```python
from build123d import *

# Parameters (mm, degrees)
SKETCH1_W               = 34.29
SKETCH1_H               = 25.4
BOSS_EXTRUDE1_DEPTH     = 2.54
SKETCH3_W               = 49.53
SKETCH3_H               = 6.35
BOSS_EXTRUDE2_DEPTH     = 3.81
CUT_EXTRUDE1_DEPTH      = 50.415894204
CUT_EXTRUDE1_DEPTH_BACK = 50.415894204
SKETCH2_R               = 1.778
SKETCH5_W               = 7.62
SKETCH5_H               = 6.35
BOSS_EXTRUDE3_DEPTH     = 15.24
BOSS_EXTRUDE4_REACH     = 53.321
SKETCH6_W               = 7.62
SKETCH6_H               = 5.08
SKETCH7_R               = 2.04
SKETCH7_R_2             = 2.039999984
CUT_EXTRUDE2_DEPTH      = 53.578613523
SKETCH9_W               = 2.794
SKETCH9_H               = 12.699691263
CUT_EXTRUDE3_DEPTH      = 58.711684259


with BuildPart() as part:
    # Sketch1 → Boss-Extrude1 (new body)
    with BuildSketch(Plane.XY):
        with Locations((17.145, 12.7)):
            Rectangle(SKETCH1_W, SKETCH1_H)
    extrude(amount=BOSS_EXTRUDE1_DEPTH)

    # Sketch3 → Boss-Extrude2 (add)
    with BuildSketch(Plane(origin=(0, 0, 0), x_dir=(-1, 0, 0), z_dir=(0, 0, -1))):
        with Locations((-17.145, 22.225)):
            Rectangle(SKETCH3_W, SKETCH3_H)
        with Locations((-17.145, 3.175)):
            Rectangle(SKETCH3_W, SKETCH3_H)
    extrude(amount=BOSS_EXTRUDE2_DEPTH)

    # Sketch2 → Cut-Extrude1 (cut, two sides: drawn at the far end of the back side and taken through both)
    with BuildSketch(Plane.XY.offset(2.54).offset(-CUT_EXTRUDE1_DEPTH_BACK)):
        with Locations((3.429, 22.606)):
            Circle(SKETCH2_R)
        with Locations((29.845, 22.86)):
            Circle(SKETCH2_R)
        with Locations((3.429, 2.794)):
            Circle(SKETCH2_R)
        with Locations((29.845, 2.286)):
            Circle(SKETCH2_R)
    extrude(amount=CUT_EXTRUDE1_DEPTH + CUT_EXTRUDE1_DEPTH_BACK, mode=Mode.SUBTRACT)

    # Sketch5 → Boss-Extrude3 (add)
    with BuildSketch(Plane.XY):
        with Locations((-3.81, 22.225)):
            Rectangle(SKETCH5_W, SKETCH5_H)
        with Locations((38.1, 22.225)):
            Rectangle(SKETCH5_W, SKETCH5_H)
        with Locations((38.1, 3.175)):
            Rectangle(SKETCH5_W, SKETCH5_H)
        with Locations((-3.81, 3.175)):
            Rectangle(SKETCH5_W, SKETCH5_H)
    extrude(amount=BOSS_EXTRUDE3_DEPTH)

    # Sketch6 → Boss-Extrude4 (add, up to next)
    with BuildSketch(Plane.XZ, mode=Mode.PRIVATE) as boss_extrude4_sk1:
        with Locations((-3.81, 12.7)):
            Rectangle(SKETCH6_W, SKETCH6_H)
    boss_extrude4_tool1 = extrude(boss_extrude4_sk1.sketch, amount=-BOSS_EXTRUDE4_REACH, mode=Mode.PRIVATE) - part.part
    # Sketch6 → Boss-Extrude4 (add, up to next)
    with BuildSketch(Plane.XZ, mode=Mode.PRIVATE) as boss_extrude4_sk2:
        with Locations((38.1, 12.7)):
            Rectangle(SKETCH6_W, SKETCH6_H)
    boss_extrude4_tool2 = extrude(boss_extrude4_sk2.sketch, amount=-BOSS_EXTRUDE4_REACH, mode=Mode.PRIVATE) - part.part
    add(boss_extrude4_tool1.solids().sort_by_distance((-3.81, 0, 12.7))[0])
    add(boss_extrude4_tool2.solids().sort_by_distance((38.1, 0, 12.7))[0])

    # Sketch7 → Cut-Extrude2 (cut, through all)
    with BuildSketch(Plane.XY.offset(15.24)):
        with Locations((38.1, 3.81)):
            Circle(SKETCH7_R)
        with Locations((38.1, 21.59)):
            Circle(SKETCH7_R_2)
        with Locations((-3.81, 3.81)):
            Circle(SKETCH7_R_2)
        with Locations((-3.81, 21.59)):
            Circle(SKETCH7_R_2)
    extrude(amount=-CUT_EXTRUDE2_DEPTH, mode=Mode.SUBTRACT)

    # Sketch9 → Cut-Extrude3 (cut, through all)
    with BuildSketch(Plane.ZY.offset(7.62)):
        with Locations((11.557, 12.700154369)):
            Rectangle(SKETCH9_W, SKETCH9_H)
    extrude(amount=-CUT_EXTRUDE3_DEPTH, mode=Mode.SUBTRACT)


solid = part.part
```
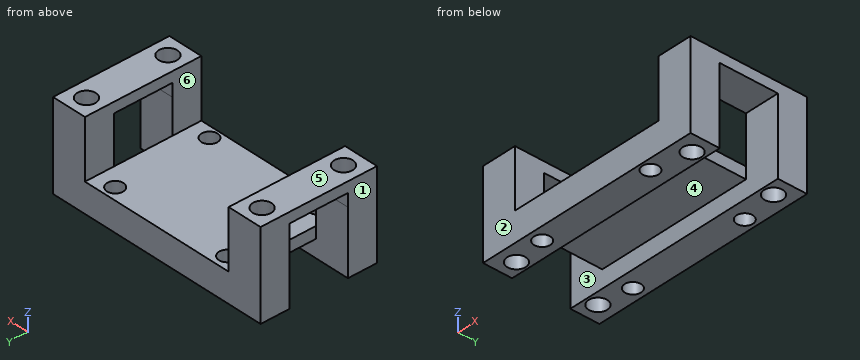
Check sheet for the modelled part. Datum: model origin and axes. Units: mm. Face numbers are marked on the shaded views. A direction names the side the tool comes from. Give positions to 0.01 mm unless a question says otherwise; leave off trailing zeros. Order: outer loops, then holes, each group sorted by start corner. A loop starts at its lowest first (then second) coordinate and runs counter-clockwise, first axis right, second up. Notation, with made-up numbers: (14, 75.25) -> (44, 75.25) arc R12 cw to (44, 79.25) -> close; hole circle Ø5 at (0.5, 84). An arc over 180 degrees is marked (long way). Return JSON: item names as keys, results as strings.
1. Go/stop test with flat-tipped pins: P1, Ø3, axis at y = 14, z = 1, coming from the +X side; P2, Ø0.8, axis at y = 10, z = 1, coming from the -X side; P3, Ø8, axis at x = 20, y = 7.5, coming from the +Z side. Record where each tip stops, or that it passes through.
From the geometry:
{"P1": "x = 34.29", "P2": "x = 0", "P3": "z = 2.54"}
2. Cross-section at B-B, the plane x = -3.81. Count the separate pieces of the cut face and the enclosed holes in it, plus the area to 3 significant figures.
From the geometry:
{"separate pieces": "3", "enclosed holes": "0", "area": "116 mm^2"}
3. Cross-section at C-C, the plane y = 17.75. Record the cut outline in (x, z).
From the geometry:
{"outline": "(-7.62, 12.95) -> (0, 12.95) -> (0, 15.24) -> (-7.62, 15.24) -> close; (0, 0) -> (34.29, 0) -> (34.29, 2.54) -> (0, 2.54) -> close; (34.29, 12.95) -> (41.91, 12.95) -> (41.91, 15.24) -> (34.29, 15.24) -> close"}
4. Mould release check, pull along Y, two halves, no side actions. Record for the marked faces 1, 2 and 3: +Y half, -Y half, draft (parallel to the pull), parting line (faces both ways), or undercut.
From the geometry:
{"face 1": "draft", "face 2": "-Y half", "face 3": "undercut"}
5. Set-up check for the marked faces 4, 5 and 6: record each of +Z, -Z, +X, -X, +Y, -Y from which the full face is reachable in a straight line by a thin tool's end or side.
From the geometry:
{"face 4": "-Z, +X, -X", "face 5": "+Z, +X, -X, +Y, -Y", "face 6": "+Z, +Y, -Y"}
6. Material ranges on probe 1 along Y at (x, z) = (-3.81, 6.75); probe 2 along X at (y, z) = (23.75, 14.25); probe 3 along Y at (x, z) = (22.5, -1), recorded low to high. Write a range as [from, to].
From the geometry:
{"probe 1": "[0, 1.77], [5.85, 6.35], [19.05, 19.55], [23.63, 25.4]", "probe 2": "[-7.62, 0], [34.29, 41.91]", "probe 3": "[0, 6.35], [19.05, 25.4]"}
7. Cross-section at A-A, the plane z = 3.25. Record the cut outline in (x, y).
From the geometry:
{"outline": "(-7.62, 0) -> (0, 0) -> (0, 6.35) -> (-7.62, 6.35) -> close; (-7.62, 19.05) -> (0, 19.05) -> (0, 25.4) -> (-7.62, 25.4) -> close; (34.29, 0) -> (41.91, 0) -> (41.91, 6.35) -> (34.29, 6.35) -> close; (34.29, 19.05) -> (41.91, 19.05) -> (41.91, 25.4) -> (34.29, 25.4) -> close; hole circle Ø4.08 at (-3.81, 3.81); hole circle Ø4.08 at (-3.81, 21.59); hole circle Ø4.08 at (38.1, 3.81); hole circle Ø4.08 at (38.1, 21.59)"}
8. Cross-section at D-D, the plane y = 21.59. Record the cut outline in (x, z), plus the area to 3 significant figures.
From the geometry:
{"outline": "(-7.62, -3.81) -> (-5.85, -3.81) -> (-5.85, 15.24) -> (-7.62, 15.24) -> close; (-1.77, -3.81) -> (1.97, -3.81) -> (1.97, 2.54) -> (0, 2.54) -> (0, 15.24) -> (-1.77, 15.24) -> close; (4.89, -3.81) -> (28.6, -3.81) -> (28.6, 2.54) -> (4.89, 2.54) -> close; (31.09, -3.81) -> (36.06, -3.81) -> (36.06, 15.24) -> (34.29, 15.24) -> (34.29, 2.54) -> (31.09, 2.54) -> close; (40.14, -3.81) -> (41.91, -3.81) -> (41.91, 15.24) -> (40.14, 15.24) -> close", "area": "318 mm^2"}
